Could you check a few things on this model? Use its own coordinates, in mm. Face numbers are marked on the shaded views. Coordinates: 2 decimals unless noted, no trailing zeros. Loops run counter-clockwise (first coordinate to the right, second up) from the corner with the lowest first, then second, coordinate; pieces in that order, holes last. Notation, with made-up numbers: M -17,32 L -3,32 A8 ccw -3,36 Z; hole C -22.75,31 d11. An arc over 180 degrees is marked long. Write each question's results on one line, items separated by ' | '.
```python
from build123d import *
from build123d import SkipClean  # not in build123d's __all__

# Parameters (mm, degrees)
F5_DEPTH         = 1.27
F5_COPIES2_COUNT = 2
F7_R             = 3.81
F8_DEPTH         = 25.4
F9_R             = 2.54
F10_DEPTH        = 25.4
F9_R_2           = 40.64
F9_W             = 8.89
F9_H             = 1.27
F9_R_3           = 19.05
F11_DEPTH        = 2.54
F12_R            = 48.26
F12_R_2          = 40.64
F13_DEPTH        = 5.08
F15_DEPTH        = 270.51


# Not quite as in the source:
# - after a boolean that leaves OpenCascade's solid faulty, fix() repairs it
# - a pattern or mirror of a feature is missing from the dataset's text; its kind, count and spacing are read off the source's solid


with BuildPart() as f1:
    # F0 (on Front) → F1 (revolve)
    with BuildSketch(Plane.XZ):
        Polygon((-270.51, 0), (0, 0), (0, 7.62), (-57.912, 7.62), (-57.912, 12.7), (-59.69, 12.7), (-59.69, 20.32), (-63.5, 20.32), (-63.5, 48.26), (-226.06, 48.26), (-226.06, 19.05), (-229.87, 19.05), (-229.87, 7.62), (-270.51, 7.62), align=None)
    revolve(axis=Axis((-130.6665660813, 0, 0), (1, 0, 0)))

    # F4 (on offset) → F5 (join)
    with BuildSketch(Plane.XY.offset(34.925)):
        with BuildLine():
            Line((-226.06, 0), (-226.06, 4.445))
            Line((-226.06, 4.445), (-234.95, 4.445))
            Line((-234.95, 4.445), (-234.95, 3.556))
            Line((-234.95, 3.556), (-251.714, 3.556))
            ThreePointArc((-251.714, 3.556), (-254.2284717139, 2.5144717139), (-255.27, 0))
            Line((-255.27, 0), (-253.492, 0))
            ThreePointArc((-253.492, 0), (-251.714, 1.778), (-249.936, 0))
            Line((-249.936, 0), (-226.06, 0))
        make_face()
    f5 = extrude(amount=-F5_DEPTH)

    # F5_copies: F5 across plane
    add(f5.mirror(Plane(origin=(0, 0, 0), x_dir=(-1, 0, 0), z_dir=(0, 0, -1))), clean=False)

    # F5_copies1: F5 across plane
    with SkipClean():  # cleaning this boolean's faces spoils the solid; the shape is the same uncleaned
        add(f5.mirror(Plane(origin=(0, 0, 0), x_dir=(0, 0, -1), z_dir=(0, -1, 0))), clean=False)

    # F5_copies2: F5 ×2 about axis
    f5_copies2_axis = Axis((0, 0, 0), (1, 0, 0))
    with SkipClean():  # cleaning this boolean's faces spoils the solid; the shape is the same uncleaned
        for i in range(1, F5_COPIES2_COUNT):
            add(f5.rotate(f5_copies2_axis, i * 360 / F5_COPIES2_COUNT), clean=False)

    # F7 (on offset) → F8 (cut)
    with BuildSketch(Plane.XY.offset(48.26)):
        with Locations((-144.78, 0)):
            Circle(F7_R)
    extrude(amount=-F8_DEPTH, mode=Mode.SUBTRACT)

    # F9 (on face) → F10 (cut)
    with BuildSketch(Plane(origin=(-226.06, 0, 0), x_dir=(0, -1, 0), z_dir=(-1, 0, 0))):
        with Locations((30.7958633586, 17.78)):
            Circle(F9_R)
        with Locations((-30.7958633586, -17.78)):
            Circle(F9_R)
    extrude(amount=-F10_DEPTH, mode=Mode.SUBTRACT)

    # F9 (on face) → F11 (cut)
    with BuildSketch(Plane(origin=(-226.06, 0, 0), x_dir=(0, -1, 0), z_dir=(-1, 0, 0))):
        Circle(F9_R_2)
        with Locations((-30.7958633586, -17.78)):
            Circle(F9_R, mode=Mode.SUBTRACT)
        with Locations((0, -34.29)):
            Rectangle(F9_W, F9_H, mode=Mode.SUBTRACT)
        Circle(F9_R_3, mode=Mode.SUBTRACT)
        with Locations((30.7958633586, 17.78)):
            Circle(F9_R, mode=Mode.SUBTRACT)
        with Locations((0, 34.29)):
            Rectangle(F9_W, F9_H, mode=Mode.SUBTRACT)
    with SkipClean():  # cleaning this boolean's faces spoils the solid; the shape is the same uncleaned
        extrude(amount=-F11_DEPTH, mode=Mode.SUBTRACT)

    # F12 (on face) → F13 (cut)
    with BuildSketch(Plane(origin=(-226.06, 0, 0), x_dir=(0, -1, 0), z_dir=(-1, 0, 0))):
        Circle(F12_R)
        Circle(F12_R_2, mode=Mode.SUBTRACT)
    extrude(amount=-F13_DEPTH, mode=Mode.SUBTRACT)

    add(f1.part.fix(), mode=Mode.REPLACE)

    # F14 (on face) → F15 (cut, through all)
    with BuildSketch(Plane.YZ):
        with BuildLine():
            Line((5.6796126628, -5.08), (-5.6796126628, -5.08))
            ThreePointArc((-5.6796126628, -5.08), (0, -7.62), (5.6796126628, -5.08))
        make_face()
    extrude(amount=-F15_DEPTH, mode=Mode.SUBTRACT)

    add(f1.part.fix(), mode=Mode.REPLACE)


solid = f1.part
```
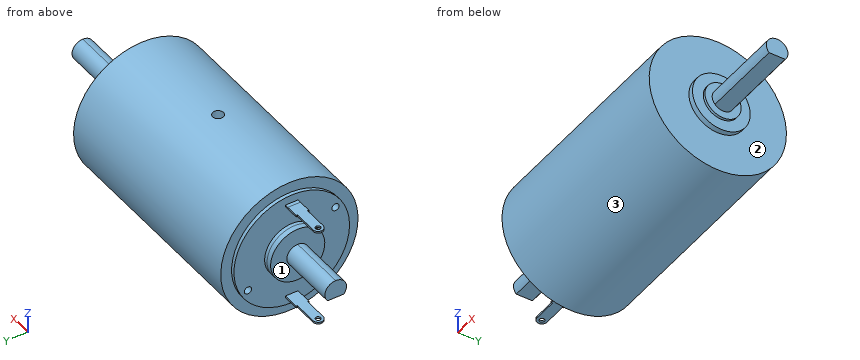
(1) Imagine slicing it at A-A, the plane x = -238. List the corners of the cut face in (y, z) for me (3 decimals).
Reported:
outline: M -5.68,-5.08 L 5.68,-5.08 A7.62 ccw long Z; M -3.556,-34.925 L 3.556,-34.925 L 3.556,-33.655 L -3.556,-33.655 Z; M -3.556,33.655 L 3.556,33.655 L 3.556,34.925 L -3.556,34.925 Z
(2) Imagine slicing it at B-B, the plane x = -144.78. List the corners of the cut face in (y, z) for me.
Reported:
outline: M -3.81,22.86 L -3.81,48.11 A48.26 ccw long 3.81,48.11 L 3.81,22.86 Z; hole M -5.68,-5.08 A7.62 ccw 5.68,-5.08 Z
(3) If we mould it in two halves opening along Z, with no side actions, what happens to the marked faces 1, 2 and 3? For each: released by +Z, released by -Z, zero draft, split by the parting line, or undercut.
Reported:
face 1: undercut | face 2: zero draft | face 3: split by the parting line
(4) Imagine slicing it at C-C, the plane z = 4.5. List the corners of the cut face in (x, y) for me, and give its area (3 significant figures).
Reported:
outline: M -270.51,-6.15 L -229.87,-6.15 L -229.87,-18.51 L -223.52,-18.51 L -223.52,-40.39 L -220.98,-40.39 L -220.98,-48.05 L -63.5,-48.05 L -63.5,-19.82 L -59.69,-19.82 L -59.69,-11.88 L -57.91,-11.88 L -57.91,-6.15 L 0,-6.15 L 0,6.15 L -57.91,6.15 L -57.91,11.88 L -59.69,11.88 L -59.69,19.82 L -63.5,19.82 L -63.5,48.05 L -220.98,48.05 L -220.98,40.39 L -223.52,40.39 L -223.52,18.51 L -229.87,18.51 L -229.87,6.15 L -270.51,6.15 Z | area: 17,000 mm2
(5) Will these pins go through, and if not, where does the flat tip stop? P1, Ø10, axis at x = -246.5, y = 1, coming from the -Z side (3 decimals); P2, Ø2, axis at x = -145, z = 33, coming from the +Y side; P3, Ø1, axis at x = -89.5, z = 7, coming from the -Y side.
Reported:
P1: stops at z = -34.925 | P2: stops at y = 36.13 | P3: stops at y = -47.82
(6) Please list where these lines run through material, in increasing order: probe 1 along X at (y, z) = (0, -34); probe 2 along X at (y, z) = (0, 30.5); probe 3 along X at (y, z) = (-32.5, 2.5). Write a range as from..to.
Reported:
probe 1: x = -255.27..-253.49, -249.94..-63.5 | probe 2: x = -223.52..-148.59, -140.97..-63.5 | probe 3: x = -223.52..-63.5
